Here's the drawing with two shaded views (mm, measured from the low corner). I have some questions. A direction names the side the tool comes from. Give positions to 0.01 mm unless a question says otherwise; leave off trailing zeros. Write each loop counter-clockwise with the first axis right and the second up, starting at its lowest first coordinate (ties: lowest second). Pieces come first, ordered by that corner, then holes.
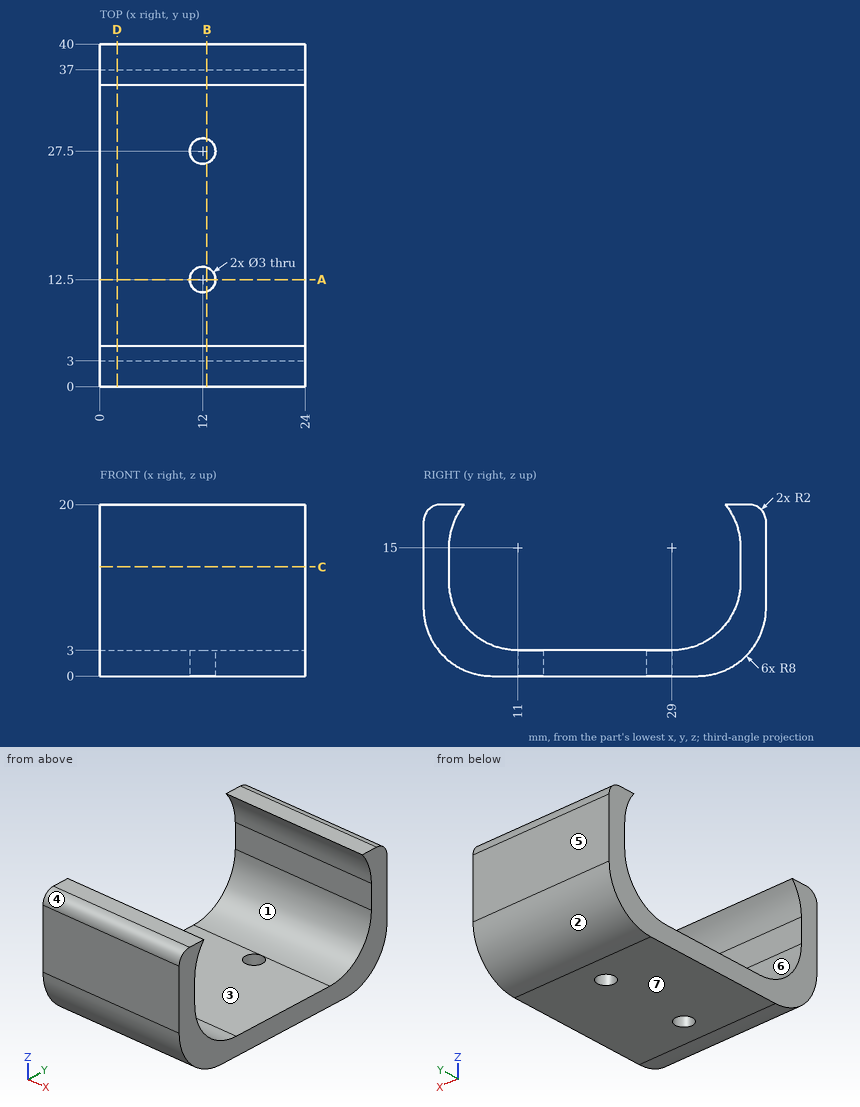
(1) If I drill on L1, parallel to Y at x = 3, z = 10.75; L2, parallel to Y at x = 12, z = 2; L3, parallel to Y at x = 12, z = 1.3, over which ranges is the centre line in solid material (lowest first)?
Returned:
L1: y = 0 to 3, 37 to 40
L2: y = 2.71 to 11, 14 to 26, 29 to 37.29
L3: y = 3.63 to 11, 14 to 26, 29 to 36.37
(2) Imagine slicing it at D-D, the plane x = 2. Write out the boundary of the cut face in (y, z) (3 decimals), plus the area to 3 significant figures.
Returned:
outline: (0, 8) arc R8 ccw to (8, 0) - (32, 0) arc R8 ccw to (40, 8) - (40, 18) arc R2 ccw to (38, 20) - (35.245, 20) arc R8 cw to (37, 15) - (37, 11) arc R8 cw to (29, 3) - (11, 3) arc R8 cw to (3, 11) - (3, 15) arc R8 cw to (4.755, 20) - (2, 20) arc R2 ccw to (0, 18) - close
area: 226 mm2
(3) Will these pins go through, and if not, where does the flat tip stop? P1, Ø1.5, axis at x = 10.5, y = 17, coming from the +Z side; P2, Ø6, axis at x = 17, y = 4.5, coming from the -Z side; P3, Ø1, axis at x = 17.5, y = 10.5, coming from the +Z side; P4, Ø2.5, axis at x = 12, y = 12.5, coming from the +Z side.
Returned:
P1: stops at z = 3
P2: stops at z = 0.02
P3: stops at z = 3.06
P4: passes through
(4) If we mould it in two halves opening along Z, with no side actions, what happens to the marked faces 4, 5, 6 and 7? For each: +Z half, -Z half, draft (parallel to the pull), parting line (faces both ways), or undercut.
Returned:
face 4: +Z half
face 5: draft
face 6: undercut
face 7: -Z half
(5) Imagine slicing it at C-C, the plane z = 12.75. Write out the boundary of the cut face in (x, y), plus the area to 3 significant figures.
Returned:
outline: (0, 0) - (24, 0) - (24, 3) - (0, 3) - close; (0, 37) - (24, 37) - (24, 40) - (0, 40) - close
area: 144 mm2
(6) For the marked faces 1, 2 and 3, which set-ups out of +Z, -Z, +X, -X, +Y, -Y let a thin tool reach every point of the face, with its end or its side?
Returned:
face 1: +X, -X
face 2: -Z, +X, -X, +Y
face 3: +Z, +X, -X
(7) Imagine slicing it at A-A, the plane y = 12.5. Write out the boundary of the cut face in (x, z).
Returned:
outline: (0, 0) - (10.5, 0) - (10.5, 3) - (0, 3) - close; (13.5, 0) - (24, 0) - (24, 3) - (13.5, 3) - close
(8) Imagine slicing it at B-B, the plane x = 12.5. Write out the boundary of the cut face in (y, z) (3 decimals), plus the area to 3 significant figures.
Returned:
outline: (0, 8) arc R8 ccw to (8, 0) - (11.086, 0) - (11.086, 3) - (11, 3) arc R8 cw to (3, 11) - (3, 15) arc R8 cw to (4.755, 20) - (2, 20) arc R2 ccw to (0, 18) - close; (13.914, 0) - (26.086, 0) - (26.086, 3) - (13.914, 3) - close; (28.914, 0) - (32, 0) arc R8 ccw to (40, 8) - (40, 18) arc R2 ccw to (38, 20) - (35.245, 20) arc R8 cw to (37, 15) - (37, 11) arc R8 cw to (29, 3) - (28.914, 3) - close
area: 209 mm2
